Geometry check sheet. Reference: the model listing, model coordinates, mm. A direction names the side the tool comes from. Give positions to 0.01 mm unless a question says otherwise; leave off trailing zeros. Loops run counter-clockwise (first coordinate to the right, second up) from the corner with the lowest first, then second, coordinate; pieces in that order, holes last.
1. Cross-section at D-D, the plane x = 183. Record the cut outline in (y, z), plus the area to 3 significant figures.
2. Cross-section at A-A, the plane z = -50. Record the cut outline in (x, y), plus the area to 3 significant figures.
3. Cross-section at C-C, the plane y = 78.5. Record the cut outline in (x, z), plus the area to 3 significant figures.
4. Tool access check on faces 4 (the cylindrical face through (1.97, 17.15, -113.51)), 5 (the cylindrical face through (201.414, 118.598, -157.173)), 6 (the flat face through (10, 34, -140.5)), 7 (the flat face through (77, 105, -131.5)), 8 (the flat face through (191.48, 106.4, -153.19)). Record the directions out of +Z, -Z, +X, -X, +Y, -Y that give a thin tool (end or side, any length) a straight path to the whole face; none if there is none.
5. Cross-section at B-B, the plane x = 55. Record the cut outline in (y, z), plus the area to 3 significant figures.
6. Material ranges on L1, parallel to Y at x = 2, z = -50; L2, parallel to Z at x = 40, y = 82; L3, parallel to X at y = 38.5, z = -123, recorded low to high.
7. Release check for a two-part mould opening along Z. For faces 1 (the flat face through (201, 121, -143.5)), 2 (the flat face through (195.17, 103.535, -155.603)), 3 (the cylindrical face through (2.028, 51.859, -47.973)) record: +Z half, -Z half, draft (parallel to the pull), parting line (faces both ways), or undercut.
8. Go/stop test with flat-tipped pins: pin 1 Ø1.2 at (x, z) = (53.5, -130.5) entering from -Y; pin 2 Ø22 at (x, y) = (77, 105.5) entering from -Z; pin 3 Ø3 at (x, z) = (2.5, -90.5) entering from +Y; pin 4 Ø4 at (y, z) = (81, -124.5) entering from -X. Record where each tip stops, or that it passes through.
from build123d import *

# Parameters (mm, degrees)
SKETCH_1_W          = 165.5
SKETCH_1_H          = 60
EXTRUDE_1_DEPTH     = 4
EXTRUDE_2_DEPTH     = 4
SKETCH_3_W          = 214.285714285
SKETCH_3_H          = 25
EXTRUDE_5_DEPTH     = 4
SKETCH_4_R          = 2.75
CUT_EXTRUDE_1_DEPTH = 4
SKETCH_5_W          = 55
SKETCH_5_H          = 20
CUT_EXTRUDE_2_DEPTH = 4
FILLET_1_R          = 10
SKETCH_6_W          = 186.285714285
SKETCH_6_H          = 14
CUT_EXTRUDE_3_DEPTH = 4
SKETCH_7_R          = 1.5
CUT_EXTRUDE_4_DEPTH = 4
FILLET_2_R          = 3
CUT_EXTRUDE_5_DEPTH = 293.240221501
CUT_EXTRUDE_6_DEPTH = 10
SKETCH_11_W         = 207.248718004
SKETCH_11_H         = 34
EXTRUDE_6_DEPTH     = 4
EXTRUDE_7_DEPTH     = 4
FILLET_3_R          = 10
CUT_EXTRUDE_7_DEPTH = 4
SKETCH_15_W         = 22
SKETCH_15_H         = 28
EXTRUDE_8_DEPTH     = 4
SKETCH_16_R         = 2.75
CUT_EXTRUDE_8_DEPTH = 10
CHAMFER_1_SIZE      = 0.5


with BuildPart() as part:
    # 草图1 → 凸台-拉伸1 (new body)
    with BuildSketch(Plane(origin=(0, 0, 0), x_dir=(0, 0, -1), z_dir=(1, 0, 0))):
        with Locations((82.75, 30)):
            Rectangle(SKETCH_1_W, SKETCH_1_H)
    extrude(amount=EXTRUDE_1_DEPTH)

    # 草图2 → 凸台-拉伸2 (add)
    with BuildSketch(Plane(origin=(0, 0, -165.5), x_dir=(-1, 0, 0), z_dir=(0, 0, -1))):
        Polygon((-4, 30), (-204, 106.930925816), (-193.94769236, 133.06425915), (-4, 60), align=None)
    extrude(amount=-EXTRUDE_2_DEPTH)

    # 草图3 → 凸台-拉伸5 (add)
    with BuildSketch(Plane(origin=(-9.536752084, 24.793025648, 0), x_dir=(0.9333333333333335, 0.3590109871422999, 0), z_dir=(0.3590109871422999, -0.9333333333333335, 0))):
        with Locations((121.646520091, -153)):
            Rectangle(SKETCH_3_W, SKETCH_3_H)
    extrude(amount=-EXTRUDE_5_DEPTH)

    # 草图4 → 切除-拉伸1 (cut)
    with BuildSketch(Plane(origin=(4, 0, 0), x_dir=(0, 0, -1), z_dir=(1, 0, 0))):
        with Locations((50, 50)):
            Circle(SKETCH_4_R)
        with Locations((50, 20)):
            Circle(SKETCH_4_R)
    extrude(amount=-CUT_EXTRUDE_1_DEPTH, mode=Mode.SUBTRACT)

    # 草图5 → 切除-拉伸2 (cut)
    with BuildSketch(Plane(origin=(4, 0, 0), x_dir=(0, 0, -1), z_dir=(1, 0, 0))):
        with Locations((138, 10)):
            Rectangle(SKETCH_5_W, SKETCH_5_H)
    extrude(amount=-CUT_EXTRUDE_2_DEPTH, mode=Mode.SUBTRACT)

    # 圆角1
    fillet_1_edges = [part.edges().sort_by_distance(p)[0] for p in [
        (2, 20, -165.5),
        (2, 20, -110.5),
        (2, 0, -110.5),
    ]]
    fillet(fillet_1_edges, radius=FILLET_1_R - 0.0001)  # a hair under: the kernel refuses the full size

    # 草图6 → 切除-拉伸3 (cut)
    with BuildSketch(Plane(origin=(-9.536752084, 24.793025648, 0), x_dir=(0.9333333333333335, 0.35901098714229984, 0), z_dir=(0.35901098714229984, -0.9333333333333335, 0))):
        with Locations((121.646520091, -147.5)):
            Rectangle(SKETCH_6_W, SKETCH_6_H)
    extrude(amount=-CUT_EXTRUDE_3_DEPTH, mode=Mode.SUBTRACT)

    # 草图7 → 切除-拉伸4 (cut)
    with BuildSketch(Plane(origin=(-9.536752084, 24.793025648, 0), x_dir=(0.9333333333333335, 0.35901098714229984, 0), z_dir=(0.35901098714229984, -0.9333333333333335, 0))):
        with Locations((221.789377233, -145.5)):
            Circle(SKETCH_7_R)
        with Locations((21.789377233, -145.5)):
            Circle(SKETCH_7_R)
    extrude(amount=-CUT_EXTRUDE_4_DEPTH, mode=Mode.SUBTRACT)

    # 圆角2
    fillet_2_edges = [part.edges().sort_by_distance(p)[0] for p in [
        (4, 32.142857143, -140.5),
        (203.281978026, 108.797592483, -140.5),
        (16.348644692, 36.892820487, -140.5),
        (190.215311359, 103.771438663, -140.5),
    ]]
    fillet(fillet_2_edges, radius=FILLET_2_R)

    # 草图8 → 切除-拉伸5 (cut, through all)
    with BuildSketch(Plane.XY.offset(-161.5)):
        Polygon((45.333333333, 45.899058002), (39.948168526, 59.899058002), (170.614835193, 110.160596202), (176, 96.160596202), align=None)
    extrude(amount=-CUT_EXTRUDE_5_DEPTH, mode=Mode.SUBTRACT)

    # 草图9 → 切除-拉伸6 (cut)
    with BuildSketch(Plane(origin=(0, 0, -161.5), x_dir=(-1, 0, 0), z_dir=(0, 0, -1))):
        Polygon((-43.897289385, 49.632391335), (-174.563956051, 99.893929535), (-176, 96.160596202), (-45.333333333, 45.899058002), align=None)
    extrude(amount=-CUT_EXTRUDE_6_DEPTH, mode=Mode.SUBTRACT)

    # 草图11 → 凸台-拉伸6 (add)
    with BuildSketch(Plane(origin=(-19.589059724, 50.926358981, 0), x_dir=(0.9333333333333335, 0.3590109871422999, 0), z_dir=(-0.3590109871422999, 0.9333333333333335, 0))):
        with Locations((125.165018231, 148.5)):
            Rectangle(SKETCH_11_W, SKETCH_11_H)
    extrude(amount=-EXTRUDE_6_DEPTH)

    # 草图12 → 凸台-拉伸7 (add)
    with BuildSketch(Plane.XY.offset(-131.5)):
        Polygon((4, 55.714285714), (4, 60), (0, 60), (0, 133.06425915), (193.94769236, 133.06425915), (195.383736309, 129.330925816), align=None)
    extrude(amount=EXTRUDE_7_DEPTH)

    # 圆角3
    fillet_3_edges = [part.edges().sort_by_distance(p)[0] for p in [
        (0, 133.06425915, -129.5),
    ]]
    fillet(fillet_3_edges, radius=FILLET_3_R)

    # 草图14 → 切除-拉伸7 (cut)
    with BuildSketch(Plane(origin=(0, 0, -131.5), x_dir=(-1, 0, 0), z_dir=(0, 0, -1))):
        with BuildLine():
            Line((-65, 123.06425915), (-35, 123.06425915))
            ThreePointArc((-35, 123.06425915), (-33, 121.06425915), (-35, 119.06425915))
            Line((-35, 119.06425915), (-65, 119.06425915))
            ThreePointArc((-65, 119.06425915), (-67, 121.06425915), (-65, 123.06425915))
        make_face()
        with BuildLine():
            Line((-65, 115.06425915), (-35, 115.06425915))
            ThreePointArc((-35, 115.06425915), (-33, 113.06425915), (-35, 111.06425915))
            Line((-35, 111.06425915), (-65, 111.06425915))
            ThreePointArc((-65, 111.06425915), (-67, 113.06425915), (-65, 115.06425915))
        make_face()
        with BuildLine():
            Line((-65, 107.06425915), (-35, 107.06425915))
            ThreePointArc((-35, 107.06425915), (-33, 105.06425915), (-35, 103.06425915))
            Line((-35, 103.06425915), (-65, 103.06425915))
            ThreePointArc((-65, 103.06425915), (-67, 105.06425915), (-65, 107.06425915))
        make_face()
    extrude(amount=-CUT_EXTRUDE_7_DEPTH, mode=Mode.SUBTRACT)

    # 草图15 → 凸台-拉伸8 (add)
    with BuildSketch(Plane(origin=(213.536752084, 82.137900168, 0), x_dir=(0, 0, -1), z_dir=(0.9333333333333338, 0.35901098714229945, 0))):
        with Locations((154.5, 40.563956051)):
            Rectangle(SKETCH_15_W, SKETCH_15_H)
    extrude(amount=EXTRUDE_8_DEPTH)

    # 草图16 → 切除-拉伸8 (cut)
    with BuildSketch(Plane(origin=(217.270085418, 83.573944117, 0), x_dir=(0, 0, -1), z_dir=(0.9333333333333335, 0.35901098714229984, 0))):
        with Locations(Location((155.5, 40.563956051, 0), (0, 0, 90))):
            Circle(SKETCH_16_R)
    extrude(amount=-CUT_EXTRUDE_8_DEPTH, mode=Mode.SUBTRACT)

    # 倒角1
    chamfer_1_edges = [part.edges().sort_by_distance(p)[0] for p in [
        (203.694459728, 118.866969765, -155.5),
    ]]
    chamfer(chamfer_1_edges, length=CHAMFER_1_SIZE)


solid = part.part
Result:
1. outline: (98.85, -165.5) - (128.85, -165.5) - (128.85, -131.5) - (133.06, -131.5) - (133.06, -127.5) - (124.57, -127.5) - (124.57, -161.5) - (103.14, -161.5) - (103.14, -154.5) - (98.85, -154.5) - close
1. area: 313 mm2
2. outline: (0, 0) - (4, 0) - (4, 17.25) - (0, 17.25) - close; (0, 22.75) - (4, 22.75) - (4, 47.25) - (0, 47.25) - close; (0, 52.75) - (4, 52.75) - (4, 60) - (0, 60) - close
2. area: 196 mm2
3. outline: (0, -131.5) - (52.1, -131.5) - (52.1, -165.5) - (88.31, -165.5) - (88.31, -161.5) - (63.24, -161.5) - (63.24, -127.5) - (0, -127.5) - close
3. area: 732 mm2
4. face 4: -Z, +X, -X, -Y
4. face 5: none
4. face 6: +Z, +X, -Y
4. face 7: -Z, -X, +Y
4. face 8: +Z
5. outline: (65.69, -165.5) - (79.62, -165.5) - (79.62, -131.5) - (103.06, -131.5) - (103.06, -127.5) - (75.33, -127.5) - (75.33, -161.5) - (65.69, -161.5) - close; (107.06, -131.5) - (111.06, -131.5) - (111.06, -127.5) - (107.06, -127.5) - close; (115.06, -131.5) - (119.06, -131.5) - (119.06, -127.5) - (115.06, -127.5) - close; (123.06, -131.5) - (133.06, -131.5) - (133.06, -127.5) - (123.06, -127.5) - close
5. area: 367 mm2
6. L1: y = 0 to 17.25, 22.75 to 47.25, 52.75 to 60
6. L2: z = -131.5 to -127.5
6. L3: x = 0 to 4
7. face 1: +Z half
7. face 2: draft
7. face 3: undercut
8. pin 1: stops at y = 74.52
8. pin 2: stops at z = -131.5
8. pin 3: stops at y = 60
8. pin 4: passes through
